Verification items for this drawing (mm, ordinates from the low corner). A direction names the side the tool comes from. Round coordinates to 2 decimals unless told otherwise and drop trailing zeros. Loops run counter-clockwise (first coordinate to the right, second up) from the corner with the lowest first, then second, coordinate; pieces in that order, holes last. Notation, with made-up numbers: (57, 37) - (100, 37) arc R19 cw to (100, 60) - close; hole circle Ø10 at (25.25, 50.25). An arc over 180 degrees is marked (long way). Answer in a Markdown table with one row per item. Add a question column.
(1) Cross-section at B-B on y = 35.5. Enter the section's corners in (x, z).
(2) Mould release check, pull along X, two halves, no side actions. Record for the marked faces 1, 2, 3 and 4: +X half, -X half, draft (parallel to the pull), parting line (faces both ways), or undercut.
(3) Gauge pin test, flat end, axial feed: pin 1 (6 mm diameter, centred on x = 8, y = 60, fed in from +Z). Record the tip position at first contact, or that the pin passes through.
(4) Access from +Z, -Z, +X, -X, +Y, -Y to the whole of each face (thin tool, end or side, straight path). Record for the marked faces 5 and 6.
(5) Thickness scan on line 1 along X through (y, z) = (60, 12.5); line 2 along Y through (x, z) = (8, 15.5); line 3 along X through (y, z) = (20, 14.5). Record the ranges inside material, lowest first.
(6) Cross-section at D-D on z = 8.25. Enter the section's corners in (x, y).
(7) Cross-section at A-A on z = 18.75. Enter the section's corners in (x, y).
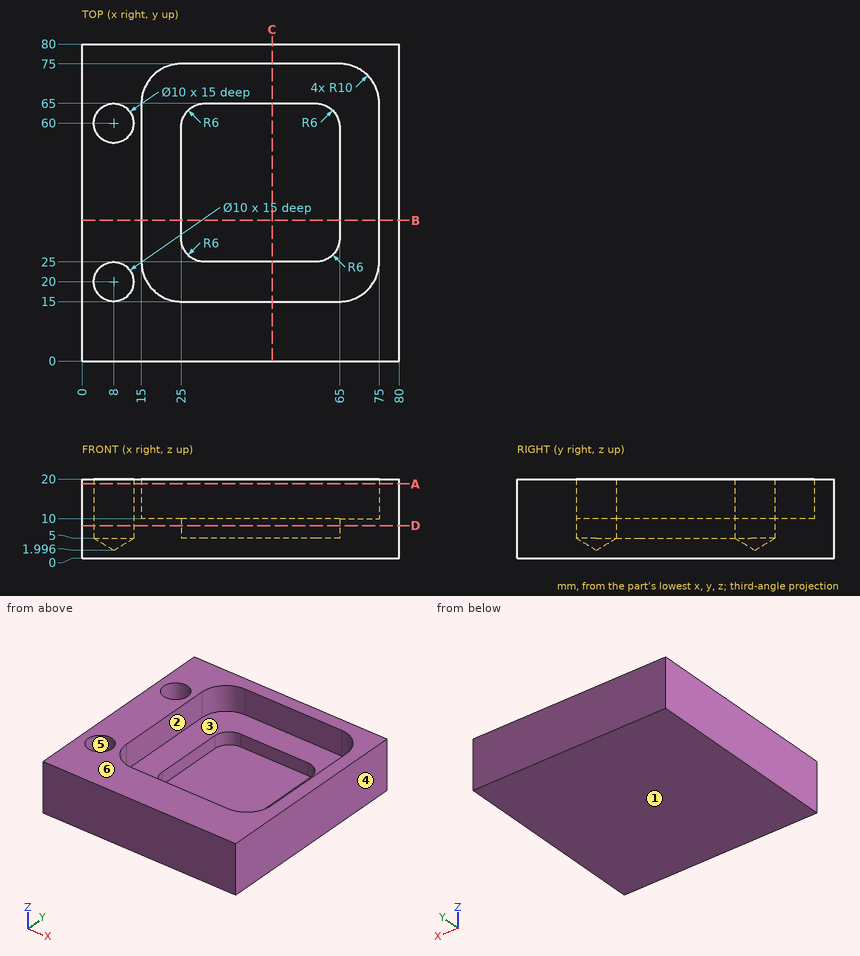
Answers:
| question | item | result |
|---|---|---|
| 1 | outline | (0, 0) - (80, 0) - (80, 20) - (75, 20) - (75, 10) - (65, 10) - (65, 5) - (25, 5) - (25, 10) - (15, 10) - (15, 20) - (0, 20) - close |
| 2 | face 1 | draft |
| 2 | face 2 | undercut |
| 2 | face 3 | undercut |
| 2 | face 4 | +X half |
| 3 | pin 1 | stops at z = 3.8 |
| 4 | face 5 | +Z |
| 4 | face 6 | +Z, +X, -X, +Y, -Y |
| 5 | line 1 | x = 0 to 3, 13 to 15, 75 to 80 |
| 5 | line 2 | y = 0 to 15, 25 to 55, 65 to 80 |
| 5 | line 3 | x = 0 to 3, 13 to 16.34, 73.66 to 80 |
| 6 | outline | (0, 0) - (80, 0) - (80, 80) - (0, 80) - close; hole circle Ø10 at (8, 20); hole circle Ø10 at (8, 60); hole (25, 31) arc R6 ccw to (31, 25) - (59, 25) arc R6 ccw to (65, 31) - (65, 59) arc R6 ccw to (59, 65) - (31, 65) arc R6 ccw to (25, 59) - close |
| 7 | outline | (0, 0) - (80, 0) - (80, 80) - (0, 80) - close; hole circle Ø10 at (8, 20); hole circle Ø10 at (8, 60); hole (15, 25) arc R10 ccw to (25, 15) - (65, 15) arc R10 ccw to (75, 25) - (75, 65) arc R10 ccw to (65, 75) - (25, 75) arc R10 ccw to (15, 65) - close |
